Input: dimensioned drawing with shaded views. Units: mm. Origin: part minimum x, y, z. Coordinates: 2 decimals unless noted, no trailing zeros. Write each loop counter-clockwise with the first axis right and the second up, starting at its lowest first coordinate (ties: lowest second). Pieces come first, ordered by that corner, then holes. Notation, with made-up numbers: (-10.5, 8) -> (26.5, 8) arc R21 cw to (26.5, 41) -> close; hole circle Ø3 at (-0.5, 43). An arc over 180 degrees is marked (long way). One line per item, written item: value. Start each with the question number.
1. Section query A-A, the plane x = 128.5. Output: boundary loops of the cut face in (y, z) (1 decimal).
2. Section query C-C, the plane x = 50. Output: boundary loops of the cut face in (y, z), and give its area (3 significant figures).
3. Line query: line 1 (X direction, y = 7.75, z = 315); line 2 (Z direction, x = 236, y = 9.5) (1 decimal); line 3 (Z direction, x = 483.5, y = 4.5) (1 decimal). Output: solid intervals per line, ascending.
4. Section query B-B, the plane z = 199. Output: boundary loops of the cut face in (x, y) (1 decimal), and give its area (3 significant figures).
5. First-contact query: P1, Ø5, axis at x = 211, y = 6, coming from the -Z side; P2, Ø4, axis at y = 5, z = 291, coming from the +X side; P3, Ø6, axis at y = 10.5, z = 476, coming from the +X side; P4, Ø7, axis at x = 484.71, z = 145.29, coming from the +Y side. Flat tips, straight axial feed; report the tip coordinate or a pass-through.
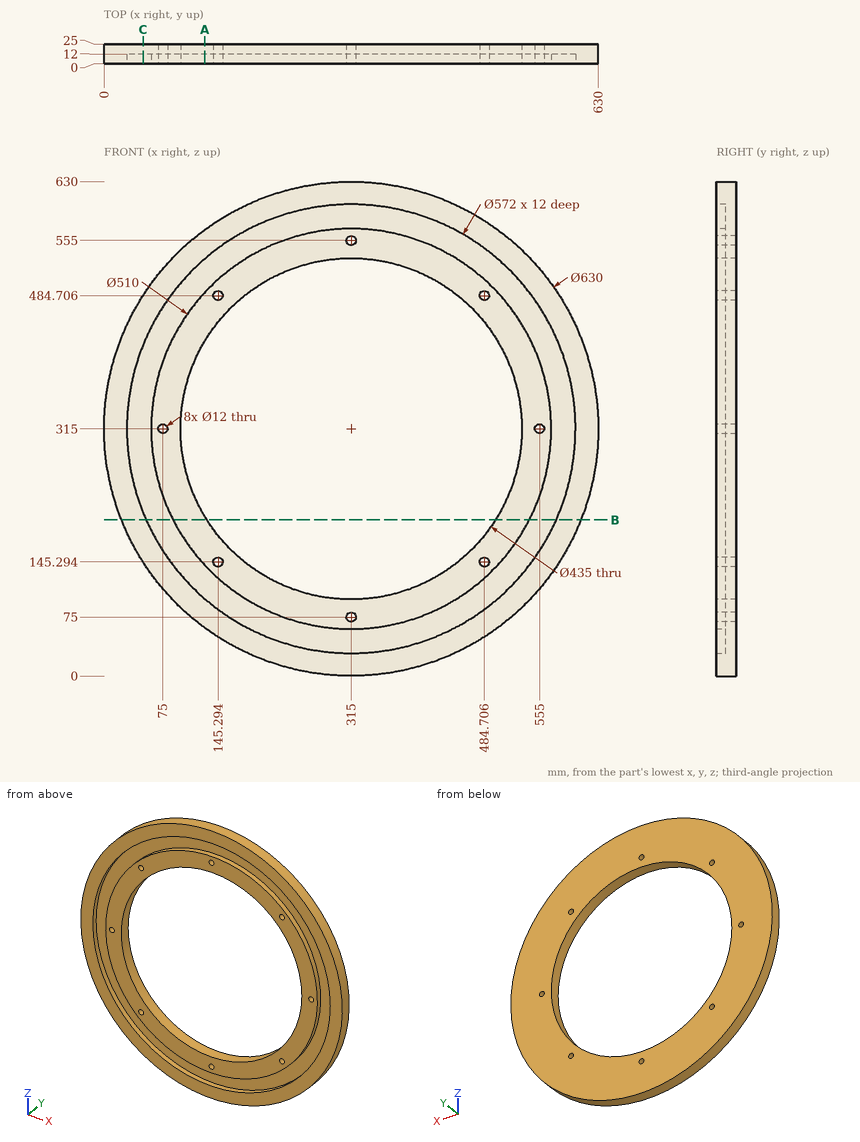
Computed values:
1. outline: (0, 61.1) -> (25, 61.1) -> (25, 203.1) -> (0, 203.1) -> (0, 141.1) -> (12, 141.1) -> (12, 98.2) -> (0, 98.2) -> close; (0, 426.9) -> (25, 426.9) -> (25, 568.9) -> (0, 568.9) -> (0, 531.8) -> (12, 531.8) -> (12, 488.9) -> (0, 488.9) -> close
2. outline: (0, 144.71) -> (25, 144.71) -> (25, 485.29) -> (0, 485.29) -> (0, 422.57) -> (12, 422.57) -> (12, 207.43) -> (0, 207.43) -> close
2. area: 5,930 mm²
3. line 1: x = 0 to 29, 60 to 69, 81 to 97.5, 532.5 to 549, 561 to 570, 601 to 630
3. line 2: z = 10.1 to 40.1, 72.5 to 112.4, 517.6 to 557.5, 589.9 to 619.9
3. line 3: z = 48.9 to 83.9, 123.6 to 139.4, 151.2 to 177.5, 452.5 to 478.8, 490.6 to 506.4, 546.1 to 581.1
4. outline: (22.1, 0) -> (53.6, 0) -> (53.6, 12) -> (87.9, 12) -> (87.9, 0) -> (131, 0) -> (131, 25) -> (22.1, 25) -> close; (499, 0) -> (542.1, 0) -> (542.1, 12) -> (576.4, 12) -> (576.4, 0) -> (607.9, 0) -> (607.9, 25) -> (499, 25) -> close
4. area: 4,620 mm²
5. P1: stops at z = 16.8
5. P2: stops at x = 629.23
5. P3: stops at x = 587.51
5. P4: passes through
